Input: part model. Units: mm. Frame: model coordinates. Face numbers are marked on the shaded views. A direction names the side the tool comes from. Coordinates: 2 decimals unless noted, no trailing zeros. Loops run counter-clockwise (first coordinate to the right, second up) from the corner with the lowest first, then second, coordinate; pieces in that order, holes last. Notation, with made-up numbers: (21.25, -10.75) - (66.25, -10.75) arc R13 ccw to (66.25, -5.75) - close; hole circle Ø2 at (67, 47). An arc over 180 degrees is marked (long way). Use a Markdown table: item, result. Add a question column.
1. Section query C-C on x = -7.5. Return the cut outline in (y, z), then the cut area to 3 significant figures.
2. Section query B-B on z = 11.5. Return the cut outline in (x, y).
3. Access query for the marked faces 1 and 2. Directions: +Z, -Z, +X, -X, +Y, -Y. A direction counts if a zero-diameter tool reaches every point of the face in a straight line with its end or side. Return the directions, or none.
4. Contact query for flat-ended pins moving along their axis: P1, Ø0.6, axis at x = 53.5, z = 3, coming from the -Y side; P2, Ø10, axis at x = -14.5, y = 24, coming from the +Z side; P3, Ø1.3, axis at x = 43.5, y = -20.5, coming from the +Z side; P4, Ø1, axis at x = 53.5, z = 6, coming from the +Y side. Output: stop coordinate, or through.
5. Draft query along Y for the marked faces 3, 4 and 5. Return one class per face: released by +Y, released by -Y, zero draft, split by the parting line, or undercut.
6. Section query D-D on y = -25.5. Return the cut outline in (x, z), then the cut area to 3 significant figures.
7. Section query A-A on y = 11.5. Return the cut outline in (x, z), then the cut area to 3 significant figures.
8. Ray query, L1, parallel to Y at x = 43.5, z = 2.75; L2, parallel to X at y = 25.5, z = 3; L3, parallel to Y at x = 22.5, z = 8. Return the intervals inside material, ascending. Write a range as [from, to].
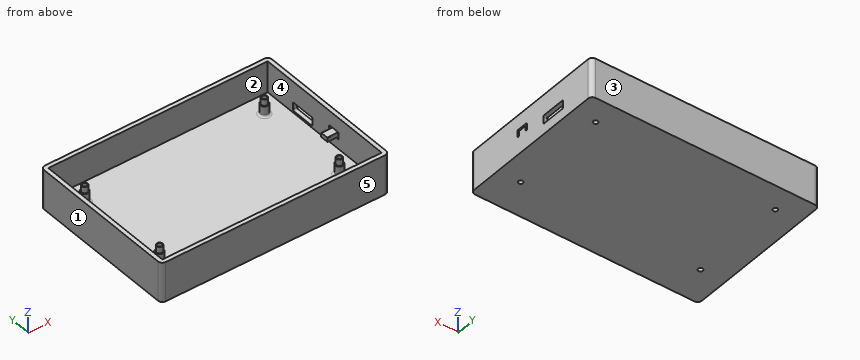
Solid Edge part; units mm, degrees
sketch "Sketch1" plane through (0, 0, 0) normal (0, 0, 1) x (1, 0, 0)
  line L0 (-54.5, -37) -> (54.5, -37)
  line L1 (54.5, -37) -> (54.5, 37)
  line L2 (54.5, 37) -> (-54.5, 37)
  line L3 (-54.5, 37) -> (-54.5, -37)
extrude "Protrusion1" add sketch "Sketch1" against normal blind 4
sketch "Sketch2" plane through (0, 0, 0) normal (0, 0, 1) x (1, 0, 0)
  line L0 (-54.5, 37) -> (-54.5, -37)
  line L1 (-54.5, -37) -> (54.5, -37)
  line L2 (54.5, -37) -> (54.5, 37)
  line L3 (54.5, 37) -> (-54.5, 37)
  line L4 (-52.5, 35) -> (-52.5, -35)
  line L5 (-52.5, -35) -> (52.5, -35)
  line L6 (52.5, -35) -> (52.5, 35)
  line L7 (52.5, 35) -> (-52.5, 35)
extrude "ExtrudedProtrusion_2" add sketch "Sketch2" along normal blind 15
sketch "Sketch3" plane through (43.5, -20.5, 5) normal (0, 0, 1) x (0, -1, 0)
  circle A0 centre (-46, -86) radius 1.4
  circle A1 centre (-46, 0) radius 1.4
  circle A2 centre (0, 0) radius 1.4
  circle A3 centre (0, -86) radius 1.4
extrude "ExtrudedProtrusion_8" add sketch "Sketch3" along normal blind 3
fillet "Round_1" radius 2 4 edges at (-54.5, -37, 5.5) (54.5, 37, 5.5) (-54.5, 37, 5.5) (54.5, -37, 5.5)
sketch "Sketch4" plane through (52.5, 0, 7.5) normal (-1, 0, 0) x (0, -1, 0)
  line L0 (-7.5, -6.5) -> (-7.5, -2.5)
  line L1 (-7.5, -2.5) -> (-19.5, -2.5)
  line L2 (-19.5, -2.5) -> (-19.5, -6.5)
  line L3 (-19.5, -6.5) -> (-7.5, -6.5)
extrude "Cutout1" cut sketch "Sketch4" against normal through all
fillet "Round1" radius 0.5 4 edges at (53.5, 7.5, 1) (53.5, 7.5, 5) (53.5, 19.5, 1) (53.5, 19.5, 5)
sketch "Sketch5" plane through (52.5, 0, 7.5) normal (-1, 0, 0) x (0, -1, 0)
  line L0 (7.5, -0.5) -> (3.5, -0.5)
  line L1 (3.5, -0.5) -> (3.5, -2.5)
  line L2 (3.5, -2.5) -> (7.5, -2.5)
  line L3 (7.5, -2.5) -> (7.5, -0.5)
extrude "ExtrudedProtrusion_9" add sketch "Sketch5" along normal blind 4.5
sketch "Sketch6" plane through (54.5, 0, 5.5) normal (1, 0, 0) x (0, 1, 0)
  arc A0 (-2.5, 1.8) -> (-3.2, 2.5) centre (-3.2, 1.8) ccw
  line L0 (-7.8008, 2.5) -> (-3.2, 2.5)
  arc A1 (-7.8008, 2.5) -> (-8.5, 1.8008) centre (-7.8008, 1.8008) ccw
  line L1 (-8.5, -0.5) -> (-8.5, 1.8008)
  line L2 (-7.5, 1.15) -> (-7.5, -0.5)
  arc A2 (-7.5, 1.15) -> (-7.15, 1.5) centre (-7.15, 1.15) cw
  line L3 (-3.8523, 1.5) -> (-7.15, 1.5)
  arc A3 (-3.8523, 1.5) -> (-3.5, 1.1477) centre (-3.8523, 1.1477) cw
  line L4 (-3.5, -0.5) -> (-3.5, 1.1477)
  line L5 (-2.5, -0.5) -> (-2.5, 1.8)
  arc A4 (-7.5, -0.5) -> (-8.5, -0.5) centre (-8, -0.5) cw
  arc A5 (-2.5, -0.5) -> (-3.5, -0.5) centre (-3, -0.5) cw
extrude "ExtrudedCutout_5" cut sketch "Sketch6" against normal blind 6.7422
sketch "Sketch7" plane through (0, 0, -4) normal (0, 0, -1) x (1, 0, 0)
  circle A0 centre (-42.5, -25.5) radius 1.9
  circle A1 centre (43.5, -25.5) radius 1.9
  circle A2 centre (43.5, 20.5) radius 1.9
  circle A3 centre (-42.5, 20.5) radius 1.9
extrude "Protrusion2" add sketch "Sketch7" against normal up to vertex (9 mm away)
sketch "Sketch8" plane through (0, 0, -4) normal (0, 0, -1) x (1, 0, 0)
  circle A0 centre (-42.5, -25.5) radius 1.1
  circle A1 centre (-42.5, 20.5) radius 1.1
  circle A2 centre (43.5, -25.5) radius 1.1
  circle A3 centre (43.5, 20.5) radius 1.1
extrude "Cutout2" cut sketch "Sketch8" against normal through all
fillet "Round_4" radius 1 4 edges at (41.6, -20.5, 0) (-44.4, -20.5, 0) (-44.4, 25.5, 0) (41.6, 25.5, 0)
Resolved:
| question | item | result |
|---|---|---|
| 1 | outline | (-37, -4) - (37, -4) - (37, 15) - (35, 15) - (35, 0) - (-35, 0) - (-35, 15) - (-37, 15) - close |
| 1 | area | 356 mm² |
| 2 | outline | (-54.5, -35) arc R2 ccw to (-52.5, -37) - (52.5, -37) arc R2 ccw to (54.5, -35) - (54.5, 35) arc R2 ccw to (52.5, 37) - (-52.5, 37) arc R2 ccw to (-54.5, 35) - close; hole (-52.5, -35) - (52.5, -35) - (52.5, 35) - (-52.5, 35) - close |
| 3 | face 1 | +Z, -Z, -X, +Y, -Y |
| 3 | face 2 | +Z |
| 4 | P1 | y = -36.87 |
| 4 | P2 | z = 0 |
| 4 | P3 | through |
| 4 | P4 | y = 36.94 |
| 5 | face 3 | released by +Y |
| 5 | face 4 | undercut |
| 5 | face 5 | released by -Y |
| 6 | outline | (-54.5, -4) - (54.5, -4) - (54.5, 15) - (52.5, 15) - (52.5, 0) - (-52.5, 0) - (-52.5, 15) - (-54.5, 15) - close |
| 6 | area | 496 mm² |
| 7 | outline | (-54.5, -4) - (54.5, -4) - (54.5, 1) - (52.5, 1) - (52.5, 0) - (-52.5, 0) - (-52.5, 15) - (-54.5, 15) - close; (52.5, 5) - (54.5, 5) - (54.5, 15) - (52.5, 15) - close |
| 7 | area | 488 mm² |
| 8 | L1 | [-37, -35], [-22.4, -21.6], [-19.4, -18.6], [23.6, 24.4], [26.6, 27.4], [35, 37] |
| 8 | L2 | [-54.5, -52.5], [-44.4, -43.6], [-41.4, -40.6], [41.6, 42.4], [44.6, 45.4], [52.5, 54.5] |
| 8 | L3 | [-37, -35], [35, 37] |
